Autodesk Inventor part; units mm, degrees
ref_plane "YZ Plane" through (0, 0, 0) normal (1, 0, 0) x (0, 1, 0)
ref_plane "XZ Plane" through (0, 0, 0) normal (0, 1, 0) x (-1, 0, 0)
ref_plane "XY Plane" through (0, 0, 0) normal (0, 0, 1) x (1, 0, 0)
sketch "Sketch1" plane through (0, 0, 0) normal (0, 0, 1) x (1, 0, 0)
  line L0 (0, 15.9441) -> (0, -15.9441) construction
  line L1 (11.6084, 0) -> (-11.6084, 0) construction
  line L2 (46.4051, 40) -> (246.4051, 40)
  line L3 (246.4051, 40) -> (246.4051, -40)
  line L4 (246.4051, -40) -> (46.4051, -40)
  line L5 (46.4051, -40) -> (46.4051, 40)
  circle A0 centre (46.4051, 0) radius 40
  circle A1 centre (246.4051, 0) radius 40
  point P0 (0, 0)
  point P1 (0, 0)
  dimension "d0" = 80
  dimension "d1" = 200
extrude "Extrusion1" add sketch "Sketch1" along normal blind 30
sketch "Sketch2" plane through (0, 0, 30) normal (0, 0, 1) x (1, 0, 0)
  arc A0 (46.4051, 40) -> (46.4051, -40) centre (46.4051, 0) ccw
  circle A1 centre (46.4051, 0) radius 40
  line L0 (46.4051, -40) -> (46.4051, 40)
  line L1 (116.4051, 0) -> (76.4051, 0)
  circle A2 centre (76.4051, 0) radius 40
  line L2 (46.4051, 40) -> (76.4051, 40)
  line L3 (76.4051, -40) -> (46.4051, -40)
  point P0 (0, 0)
extrude "Extrusion2" add sketch "Sketch2" along normal blind 110
sketch "Sketch3" plane through (46.4051, -40, 0) normal (0, -1, 0) x (1, 0, 0)
  line L0 (-40, 140) -> (0, 140)
  line L1 (0, 140) -> (10, 140)
  line L2 (10, 140) -> (-81.693, 123.8321)
  line L3 (-81.693, 123.8321) -> (-81.693, 140)
  line L4 (-81.693, 140) -> (0, 140)
  point P0 (-46.4051, 0)
extrude "Extrusion3" cut sketch "Sketch3" against normal through all
properties part number "CANH TAY 2"
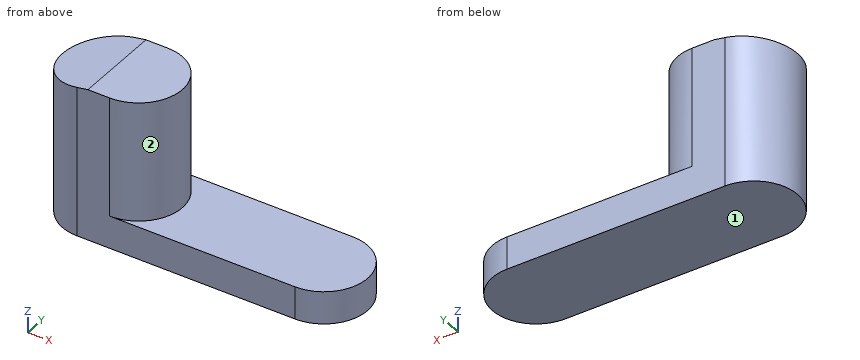
The listing builds one solid part. Answer for the finished solid, in the listing's coordinates (mm). Face numbers are marked on the shaded views. A direction names the side the tool comes from. Round coordinates to 2 decimals unless told otherwise and drop trailing zeros. Write each loop counter-clockwise with the first axis right and the second up, starting at its lowest first coordinate (ties: lowest second). Pieces come first, ordered by that corner, then holes. Notation, with made-up numbers: M -1,29.25 L 39,29.25 A10 cw 39,42.25 Z; hole C 79.25,-20.75 d9. An arc over 180 degrees is marked long. Write each question's results on one line, items separated by ' | '. Start each with the question number.
(1) The part is cut by section D-D, the plane y = 29.5. Write down the section's boundary in (x, z), and give its area (3 significant figures).
(2) For the marked faces 1 and 2, determine the directions among +Z, -Z, +X, -X, +Y, -Y from which every point of the face is accessible in a straight line to the end or side of a thin tool.
(3) The part is cut by section C-C, the plane x = 103. Write down the section's boundary in (y, z).
(4) Find the intervals of material crossed by line 1 (Z direction, x = 164.5, y = 27.5); line 2 (X direction, y = -34.5, z = 50); line 3 (X direction, y = -17, z = 28.5), in increasing order.
(5) The part is cut by section B-B, the plane z = 59.5. Write down the section's boundary in (x, y), and give its area (3 significant figures).
(6) The part is cut by section A-A, the plane y = 0. Write down the section's boundary in (x, z).
(7) Each of these flat-tipped pins is pushed along its axis until it touches: P1, Ø1.5, axis at y = 3, z = 30.5, coming from the +X side; P2, Ø8, axis at y = 13, z = 90, coming from the -X side; P3, Ø12, axis at x = 254, z = 32.5, coming from the +Y side. Where does it stop, or does it pass through?
Worked answers:
1) outline: M 19.39,0 L 273.42,0 L 273.42,30 L 103.42,30 L 103.42,140 L 56.41,140 L 19.39,133.47 Z | area: 16,700 mm²
2) face 1: -Z, +X, -X, +Y, -Y | face 2: +Z, +X
3) outline: M -40,0 L 40,0 L 40,30 L 29.88,30 L 29.88,140 L -29.88,140 L -29.88,30 L -40,30 Z
4) line 1: z = 0 to 30 | line 2: x = 26.16 to 96.65 | line 3: x = 10.2 to 282.61
5) outline: M 46.41,-40 L 76.41,-40 A40 ccw 76.41,40 L 46.41,40 A40 ccw Z | area: 7,430 mm²
6) outline: M 6.41,0 L 286.41,0 L 286.41,30 L 116.41,30 L 116.41,140 L 56.41,140 L 6.41,131.18 Z
7) P1: stops at x = 286.33 | P2: stops at x = 7.43 | P3: stops at y = 39.94
